```python
from build123d import *

# Parameters (mm, degrees)
F0_R     = 42
F0_R_2   = 40
F1_DEPTH = 15
F0_R_3   = 9.5
F0_R_4   = 7.5
F3_DEPTH = 10


with BuildPart() as f1:
    # F0 (on Top) → F1 (new body)
    with BuildSketch(Plane.XY):
        Circle(F0_R)
        Circle(F0_R_2, mode=Mode.SUBTRACT)
    extrude(amount=F1_DEPTH)



with BuildPart() as f1b:
    # F0 (on Top) → F1, piece 2 (new body)
    with BuildSketch(Plane.XY):
        Circle(F0_R_3)
        Circle(F0_R_4, mode=Mode.SUBTRACT)
    extrude(amount=F1_DEPTH)


with BuildPart() as f1_1:
    add(f1.part)

    add(f1b.part)  # F3 merges F1b
    # F2 (on Top) → F3 (join)
    with BuildSketch(Plane.XY):
        with BuildLine():
            ThreePointArc((39.9617004143, -1.75), (39.9904239573, -0.8752095261), (40, 0))
            ThreePointArc((40, 0), (39.9904239573, 0.8752095261), (39.9617004143, 1.75))
            Line((39.9617004143, 1.75), (9.3374246985, 1.75))
            ThreePointArc((9.3374246985, 1.75), (9.4592688575, 0.8787677066), (9.5, 0))
            ThreePointArc((9.5, 0), (9.4592688575, -0.8787677066), (9.3374246985, -1.75))
            Line((9.3374246985, -1.75), (39.9617004143, -1.75))
        make_face()
        with BuildLine():
            Line((-9.3374246985, 1.75), (-39.9617004143, 1.75))
            ThreePointArc((-39.9617004143, 1.75), (-40, 0), (-39.9617004143, -1.75))
            Line((-39.9617004143, -1.75), (-9.3374246985, -1.75))
            ThreePointArc((-9.3374246985, -1.75), (-9.5, 0), (-9.3374246985, 1.75))
        make_face()
    extrude(amount=F3_DEPTH)


solid = f1_1.part
```
The listing builds one solid part. Answer for the finished solid, in the listing's coordinates (mm). A direction names the side the tool comes from. Round coordinates to 2 decimals unless told otherwise and drop trailing zeros. Write each loop counter-clockwise with the first axis right and the second up, starting at its lowest first coordinate (ties: lowest second). Pieces come first, ordered by that corner, then holes. Notation, with made-up numbers: (-22, 41) -> (-1, 41) arc R20 cw to (-1, 70) -> close; hole circle Ø4 at (74, 44.25). An arc over 180 degrees is marked (long way). Use CSV: the item, a comma, the result in double quotes. Start each with the question number.
(1) The mould has two halves that part along Y. Classify faces 1 (the face through (40.06, 12.62, 7.4)), 2 (the face through (24, -1.75, 5)), 3 (the face through (37.1, -15.4, 15)), 4 (the face through (-25, 0, 10)): released by +Y, released by -Y, zero draft, split by the parting line, or undercut.
(2) Section C-C on y = 0 is taken. Give the vertices of the cut face in (x, z), then the cut area to 3 significant figures.
(3) Section B-B on z = 1.25 is taken. Give the vertices of the cut face in (x, y).
(4) Section D-D on x = 18 is taken. Give the vertices of the cut face in (y, z), then the cut area to 3 significant figures.
(5) Which of the six approach directions +Z, -Z, +X, -X, +Y, -Y give full straight-line access (tool end or side, diameter ignored) to faces 5 (the face through (24, 0, 10)), 6 (the face through (-25, -1.75, 5)), 7 (the face through (1, 8, 15))?
(6) Consider L1, parallel to Y at x = 0, z = 4.75; L2, parallel to X at y = 5, z = 4.75; L3, parallel to Y at x = 1, z = 4.5. Determine where each line is inside the solid, lowest interval first. Write a range as from..to.
(7) Section A-A on x = 0 is taken. Give the vertices of the cut face in (y, z), then the cut area to 3 significant figures.
(8) Each of these flat-tipped pins is pushed along its axis until it touches: pin 1 (2 mm diameter, centred on x = 3, z = 2.5, fed in from +Y); pin 2 (1 mm diameter, centred on y = -22.5, z = 5.5, fed in from +X); pin 3 (1.8 mm diameter, centred on x = -25, y = 0.5, fed in from +Z). Where does it stop, or does it pass through?
A:
1,face 1,"split by the parting line"
1,face 2,"undercut"
1,face 3,"zero draft"
1,face 4,"undercut"
2,outline,"(-42, 0) -> (-7.5, 0) -> (-7.5, 15) -> (-9.5, 15) -> (-9.5, 10) -> (-40, 10) -> (-40, 15) -> (-42, 15) -> close; (7.5, 0) -> (42, 0) -> (42, 15) -> (40, 15) -> (40, 10) -> (9.5, 10) -> (9.5, 15) -> (7.5, 15) -> close"
2,area,"730 mm²"
3,outline,"circle Ø84 at (0, 0); hole (-39.96, -1.75) arc R40 ccw to (39.96, -1.75) -> (9.34, -1.75) arc R9.5 cw to (-9.34, -1.75) -> close; hole (-39.96, 1.75) -> (-9.34, 1.75) arc R9.5 cw to (9.34, 1.75) -> (39.96, 1.75) arc R40 ccw to start; hole circle Ø15 at (0, 0)"
4,outline,"(-37.95, 0) -> (-35.72, 0) -> (-35.72, 15) -> (-37.95, 15) -> close; (-1.75, 0) -> (1.75, 0) -> (1.75, 10) -> (-1.75, 10) -> close; (35.72, 0) -> (37.95, 0) -> (37.95, 15) -> (35.72, 15) -> close"
4,area,"102 mm²"
5,face 5,"+Z"
5,face 6,"+Z, -Z"
5,face 7,"+Z, +X, -X, +Y, -Y"
6,L1,"y = -42..-40, -9.5..-7.5, 7.5..9.5, 40..42"
6,L2,"x = -41.7..-39.69, -8.08..-5.59, 5.59..8.08, 39.69..41.7"
6,L3,"y = -41.99..-39.99, -9.45..-7.43, 7.43..9.45, 39.99..41.99"
7,outline,"(-42, 0) -> (-40, 0) -> (-40, 15) -> (-42, 15) -> close; (-9.5, 0) -> (-7.5, 0) -> (-7.5, 15) -> (-9.5, 15) -> close; (7.5, 0) -> (9.5, 0) -> (9.5, 15) -> (7.5, 15) -> close; (40, 0) -> (42, 0) -> (42, 15) -> (40, 15) -> close"
7,area,"120 mm²"
8,pin 1,"stops at y = 41.95"
8,pin 2,"stops at x = 35.78"
8,pin 3,"stops at z = 10"
